```python
from build123d import *

# Parameters (mm, degrees)
ESTRUSIONE_ESTRUSIONE1_DEPTH = 21.54
SCHIZZO2_W                   = 21.54
SCHIZZO2_H                   = 30
SCHIZZO2_R                   = 9
TAGLIO_ESTRUSIONE1_DEPTH     = 60


with BuildPart() as part:
    # Schizzo1 → Estrusione-Estrusione1 (new body)
    with BuildSketch(Plane.XY):
        with BuildLine():
            Line((0, 15), (100, 15))
            ThreePointArc((100, 15), (107.5, 12.990381057), (112.990381057, 7.5))
            Line((112.990381057, 7.5), (109.09326674, 5.25))
            ThreePointArc((109.09326674, 5.25), (89.5, 0), (109.09326674, -5.25))
            Line((109.09326674, -5.25), (112.990381057, -7.5))
            ThreePointArc((112.990381057, -7.5), (107.5, -12.990381057), (100, -15))
            Line((100, -15), (0, -15))
            ThreePointArc((0, -15), (-7.5, -12.990381057), (-12.990381057, -7.5))
            Line((-12.990381057, -7.5), (-9.09326674, -5.25))
            ThreePointArc((-9.09326674, -5.25), (10.5, 0), (-9.09326674, 5.25))
            Line((-9.09326674, 5.25), (-12.990381057, 7.5))
            ThreePointArc((-12.990381057, 7.5), (-7.5, 12.990381057), (0, 15))
        make_face()
    extrude(amount=ESTRUSIONE_ESTRUSIONE1_DEPTH)

    # Schizzo2 → Taglio-Estrusione1 (cut)
    with BuildSketch(Plane(origin=(20, 0, 0), x_dir=(0, 0, -1), z_dir=(1, 0, 0))):
        with Locations((-10.77, 0)):
            Rectangle(SCHIZZO2_W, SCHIZZO2_H)
        with Locations((-10.77, 0)):
            Circle(SCHIZZO2_R, mode=Mode.SUBTRACT)
    extrude(amount=TAGLIO_ESTRUSIONE1_DEPTH, mode=Mode.SUBTRACT)


solid = part.part
```
Model file for the job. Use its own axes, mm. A direction names the side the tool comes from. Give positions to 0.01 mm unless a question says otherwise; leave off trailing zeros. Loops run counter-clockwise (first coordinate to the right, second up) from the corner with the lowest first, then second, coordinate; pieces in that order, holes last. Notation, with made-up numbers: (54.5, 34.5) -> (66.5, 34.5) arc R8 ccw to (66.5, 38.5) -> close; hole circle Ø2 at (-22, 75.5). An arc over 180 degrees is marked (long way). Use CSV: the item, a comma, the result in double quotes. Start each with the question number.
1) Mould opens along Y. For faces 1 (the cylindrical face through (107.595, -12.935, 10.619)), 2 (the cylindrical face through (89.507, 0.385, 10.619)), 3 (the flat face through (10, 15, 11)) say: released by +Y, released by -Y, zero draft, split by the parting line, or undercut.
2) Tool access for faces 4 (the flat face through (20, 0, 1)), 5 (the flat face through (111.015, -6.359, 10.619)), 6 (the flat face through (-11.07, -6.39, 10.62)): list every direction of +Z, -Z, +X, -X, +Y, -Y with a clear straight run to the whole face (end or side of a thin tool).
3) Slice it at A-A on y = 12. Give the cut face in (x, z), plus the area to 3 significant figures.
4) Flat gauge pins, fed straight in: pin 1 Ø6 at (x, z) = (64, 5) entering from +Y; pin 2 Ø2 at (y, z) = (3.5, 5.5) entering from -X; pin 3 Ø10 at (x, z) = (32.5, 9.5) entering from +Y. Where does each tip first touch, or does it go through?
5) Slice it at B-B on x = 5. Give the cut face in (y, z), plus the area to 3 significant figures.
6) Slice it at D-D on z = 4. Give the cut face in (x, y), plus the area to 3 significant figures.
7) Slice it at C-C on y = 0. Give the cut face in (x, z).
8) Wall check: line 1 (Y direction, x = 0, z = 10); line 2 (X direction, y = -5.5, z = 5.5); line 3 (X direction, y = 6.75, z = 1.75). Give the ranges that are in metal, low to high.
Computed values:
1,face 1,"released by -Y"
1,face 2,"undercut"
1,face 3,"released by +Y"
2,face 4,"none"
2,face 5,"+Z, -Z, +X"
2,face 6,"+Z, -Z, -X"
3,outline,"(-9, 0) -> (20, 0) -> (20, 21.54) -> (-9, 21.54) -> close; (80, 0) -> (109, 0) -> (109, 21.54) -> (80, 21.54) -> close"
3,area,"1,250 mm^2"
4,pin 1,"stops at y = 8.56"
4,pin 2,"stops at x = 9.49"
4,pin 3,"stops at y = 9"
5,outline,"(-15, 0) -> (-9.23, 0) -> (-9.23, 21.54) -> (-15, 21.54) -> close; (9.23, 0) -> (15, 0) -> (15, 21.54) -> (9.23, 21.54) -> close"
5,area,"248 mm^2"
6,outline,"(-12.99, -7.5) arc R15 ccw to (0, -15) -> (20, -15) -> (20, -5.93) -> (80, -5.93) -> (80, -15) -> (100, -15) arc R15 ccw to (112.99, -7.5) -> (109.09, -5.25) arc R10.5 cw (long way) to (109.09, 5.25) -> (112.99, 7.5) arc R15 ccw to (100, 15) -> (80, 15) -> (80, 5.93) -> (20, 5.93) -> (20, 15) -> (0, 15) arc R15 ccw to (-12.99, 7.5) -> (-9.09, 5.25) arc R10.5 cw (long way) to (-9.09, -5.25) -> close"
6,area,"1,810 mm^2"
7,outline,"(10.5, 0) -> (20, 0) -> (20, 1.77) -> (80, 1.77) -> (80, 0) -> (89.5, 0) -> (89.5, 21.54) -> (80, 21.54) -> (80, 19.77) -> (20, 19.77) -> (20, 21.54) -> (10.5, 21.54) -> close"
8,line 1,"y = -15 to -10.5, 10.5 to 15"
8,line 2,"x = -9.53 to -8.94, 8.94 to 91.06, 108.94 to 109.53"
8,line 3,"x = -11.69 to -8.04, 8.04 to 20, 80 to 91.96, 108.04 to 111.69"
